Can you work these out from the model? Positions are in its coordinate system, mm. Face numbers are marked on the shaded views. Give positions to 0.01 mm unless a question says otherwise; leave off trailing zeros. Order: outer loops, then holes, each group sorted by start corner. A loop starts at its lowest first (then second) coordinate and runs counter-clockwise, first axis right, second up. Notation, with made-up numbers: M 66,87 L 119,87 A10 ccw 119,92 Z; hole C 8,37 d4. An arc over 180 degrees is marked long. One line per question, with ' | ' between items. Start each with the question number.
1) Thinking about a two-plate mould opening in Z: for the marked faces 1, 2, 3 and 4, which applies, +Z half, -Z half, draft (parallel to the pull), parting line (faces both ways), or undercut?
2) If we section it at B-B, the plane x = 0: Please give me the cut outline in (y, z).
3) Please list where these lines run through material, in increasing order: line 1 along X through (y, z) = (-3.5, -0.5); line 2 along Y through (x, z) = (-23, 0); line 3 along X through (y, z) = (-5.5, 0). Write a range as [from, to].
4) If we section it at C-C, the plane y = 1.5: Please give me the cut outline in (x, z), plus the area to 3 significant figures.
5) If we section it at D-D, the plane x = -10: Please give me the cut outline in (y, z).
6) I'm going to push flat-ended pins straight in: pin 1 Ø3 at (x, y) = (-5, 7.5) entering from +Z; pin 2 Ø6.5 at (y, z) = (-1, 1.5) entering from -X; pin 3 Ø4 at (y, z) = (-2.5, 10) entering from +X; pin 4 Ø2.5 at (x, z) = (-24, -0.5) entering from +Y. Where does each tip first touch, or does it pass through?
7) If we section it at A-A, the plane z = 0: Please give me the cut outline in (x, y).
```python
from build123d import *

# Parameters (mm, degrees)
SKETCH_2_R          = 22.7
SKETCH_2_R_2        = 12.7
EXTRUDE_1_DEPTH     = 10
EXTRUDE_START       = -20
EXTRUDE_2_DEPTH     = 5
SKETCH_4_R          = 4
CUT_EXTRUDE_2_DEPTH = 5


with BuildPart() as part:
    # Эскиз2 → Бобышка-Вытянуть1 (new, symmetric)
    with BuildSketch(Plane(origin=(0, 0, 0), x_dir=(1, 0, 0), z_dir=(0, 1, 0))):
        with Locations(Location((0, 0, 0), (0, 0, 270))):
            Circle(SKETCH_2_R)
        with Locations(Location((0, 0, 0), (0, 0, 270))):
            Circle(SKETCH_2_R_2, mode=Mode.SUBTRACT)
    extrude(amount=EXTRUDE_1_DEPTH, both=True)

    # Эскиз3 → Бобышка-Вытянуть2 (add)
    with BuildSketch(Plane(origin=(0, 0, 0), x_dir=(0, 0, -1), z_dir=(1, 0, 0)).offset(EXTRUDE_START)):
        Polygon((5.773502692, 0), (2.886751346, 5), (-2.886751346, 5), (-5.773502692, 0), (-2.886751346, -5), (2.886751346, -5), align=None)
    extrude(amount=-EXTRUDE_2_DEPTH)

    # Эскиз4 → Вырез-Вытянуть2 (cut)
    with BuildSketch(Plane.ZY.offset(25)):
        Circle(SKETCH_4_R)
    extrude(amount=-CUT_EXTRUDE_2_DEPTH, mode=Mode.SUBTRACT)


solid = part.part
```
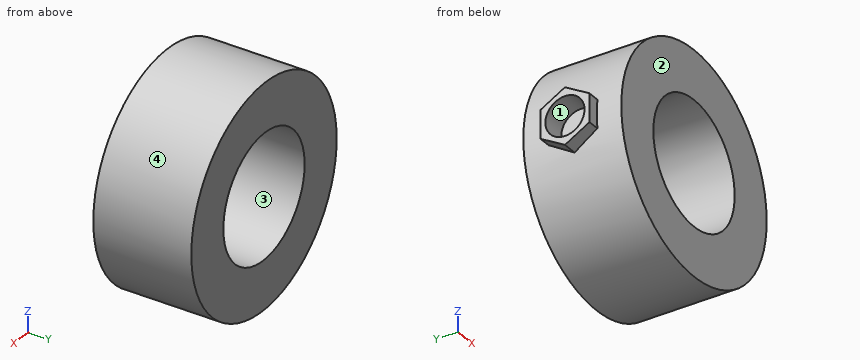
Results found:
1) face 1: undercut | face 2: draft | face 3: undercut | face 4: parting line
2) outline: M -10,-22.7 L 10,-22.7 L 10,-12.7 L -10,-12.7 Z; M -10,12.7 L 10,12.7 L 10,22.7 L -10,22.7 Z
3) line 1: x = [-20, -12.69], [12.69, 22.69] | line 2: y = [-5, -4], [4, 5] | line 3: x = [-22.7, -12.7], [12.7, 22.7]
4) outline: M -25,-4.91 L -22.16,-4.91 A22.7 ccw long -22.16,4.91 L -25,4.91 L -25,3.71 L -20,3.71 L -20,-3.71 L -25,-3.71 Z; hole C 0,0 d25.4 | area: 1,100 mm²
5) outline: M -10,-20.38 L 10,-20.38 L 10,-7.83 L -10,-7.83 Z; M -10,7.83 L 10,7.83 L 10,20.38 L -10,20.38 Z
6) pin 1: stops at z = 22.43 | pin 2: stops at x = -25 | pin 3: stops at x = 21.24 | pin 4: stops at y = 5
7) outline: M -25,-5 L -22.7,-5 L -22.7,-10 L -12.7,-10 L -12.7,10 L -22.7,10 L -22.7,5 L -25,5 L -25,4 L -20,4 L -20,-4 L -25,-4 Z; M 12.7,-10 L 22.7,-10 L 22.7,10 L 12.7,10 Z
